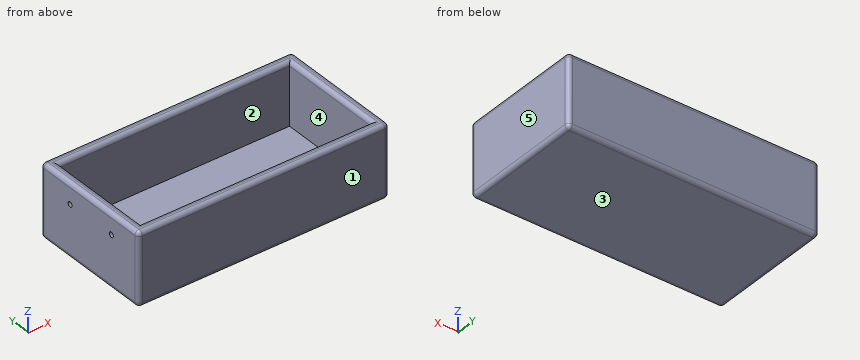
from build123d import *

# Parameters (mm, degrees)
F0_W     = 121.37
F0_H     = 60.8
F0_W_2   = 111.37
F0_H_2   = 50.8
F1_DEPTH = 5
F2_DEPTH = 35
F3_R     = 1.25
F4_DEPTH = 75
F5_R     = 2


with BuildPart() as f1:
    # F0 (on Top) → F1 (new body)
    with BuildSketch(Plane.XY):
        with Locations((-0.463949, -2.512982)):
            Rectangle(F0_W, F0_H)
        with Locations((-0.463949, -2.512982)):
            Rectangle(F0_W_2, F0_H_2, mode=Mode.SUBTRACT)
        with Locations((-0.463949, -2.512982)):
            Rectangle(F0_W_2, F0_H_2)
    extrude(amount=F1_DEPTH)

    # F0 (on Top) → F2 (join)
    with BuildSketch(Plane.XY):
        with Locations((-0.463949, -2.512982)):
            Rectangle(F0_W, F0_H)
        with Locations((-0.463949, -2.512982)):
            Rectangle(F0_W_2, F0_H_2, mode=Mode.SUBTRACT)
    extrude(amount=F2_DEPTH)

    # F3 (on Right) → F4 (cut)
    with BuildSketch(Plane.YZ):
        with Locations((-16.162982, 25.25)):
            Circle(F3_R)
        with Locations((9.637018, 25.25)):
            Circle(F3_R)
    extrude(amount=-F4_DEPTH, mode=Mode.SUBTRACT)

    # F5
    f5_edges = [f1.edges().sort_by_distance(p)[0] for p in [
        (-61.148949, -32.912982, 17.5),
        (-0.463949, -32.912982, 35),
        (60.221051, -32.912982, 17.5),
        (-0.463949, -32.912982, 0),
        (60.221051, 27.887018, 17.5),
        (-0.463949, 27.887018, 35),
        (-61.148949, 27.887018, 17.5),
        (-0.463949, 27.887018, 0),
        (60.221051, -2.512982, 35),
        (60.221051, -2.512982, 0),
        (55.221051, -2.512982, 35),
        (-0.463949, 22.887018, 35),
        (-56.148949, -2.512982, 35),
        (-0.463949, -27.912982, 35),
        (-61.148949, -2.512982, 35),
        (-61.148949, -2.512982, 0),
    ]]
    fillet(f5_edges, radius=F5_R)


solid = f1.part
The listing builds one solid part. Answer for the finished solid, in the listing's coordinates (mm). Face numbers are marked on the shaded views. A direction names the side the tool comes from. Give positions to 0.01 mm unless a question says otherwise; leave off trailing zeros. Write each loop counter-clockwise with the first axis right and the second up, starting at its lowest first coordinate (ties: lowest second). Pieces come first, ordered by that corner, then holes.
1) Given P1, Ø6, axis at x = 39.5, y = -0.5, coming from the -Z side; P2, Ø2, axis at x = -44.5, y = 0, coming from the +Z side, each flat-ended and moving along its own axis, determine where each tip first touches the part or whether it passes through.
2) Section A-A (z = 25.25) is taken. Write down the section's boundary in (x, y), and give its area (3 significant figures).
3) Find the intervals of material crossed by L1, parallel to Y at x = -58, z = 25; L2, parallel to Y at x = 12, z = 20.5; L3, parallel to X at y = -20, z = 21, in increasing order.
4) Section C-C (x = -46) is taken. Write down the section's boundary in (y, z).
5) A tool of negligible diameter and unlimited length cuts with its end or side. For the marked faces 1 and 2, from which of +Z, -Z, +X, -X, +Y, -Y can it reach the whole face along a straight path? Write none if from no direction.
6) Section B-B (y = -3.5) is taken. Write down the section's boundary in (x, z).
7) For a pull along X with two mould halves and no side action, classify the marked faces 3, 4 and 5 as pulls with the +X half, pulls with the -X half, needs draft (parallel to the pull), parting line crosses it, or undercut.
Response:
1. P1: stops at z = 0
1. P2: stops at z = 5
2. outline: (-61.15, -30.91) arc R2 ccw to (-59.15, -32.91) - (58.22, -32.91) arc R2 ccw to (60.22, -30.91) - (60.22, 25.89) arc R2 ccw to (58.22, 27.89) - (-59.15, 27.89) arc R2 ccw to (-61.15, 25.89) - (-61.15, 10.89) - (-56.15, 10.89) - (-56.15, 22.89) - (55.22, 22.89) - (55.22, -27.91) - (-56.15, -27.91) - (-56.15, -17.41) - (-61.15, -17.41) - close; (-61.15, -14.91) - (-56.15, -14.91) - (-56.15, 8.39) - (-61.15, 8.39) - close
2. area: 1,690 mm2
3. L1: y = -32.91 to -17.39, -14.94 to 8.41, 10.86 to 27.89
3. L2: y = -32.91 to -27.91, 22.89 to 27.89
3. L3: x = -61.15 to -56.15, 55.22 to 60.22
4. outline: (-32.91, 2) arc R2 ccw to (-30.91, 0) - (25.89, 0) arc R2 ccw to (27.89, 2) - (27.89, 33) arc R2 ccw to (25.89, 35) - (24.89, 35) arc R2 ccw to (22.89, 33) - (22.89, 5) - (-27.91, 5) - (-27.91, 33) arc R2 ccw to (-29.91, 35) - (-30.91, 35) arc R2 ccw to (-32.91, 33) - close
5. face 1: +Z, -Z, +X, -X, -Y
5. face 2: +Z
6. outline: (-61.15, 2) arc R2 ccw to (-59.15, 0) - (58.22, 0) arc R2 ccw to (60.22, 2) - (60.22, 33) arc R2 ccw to (58.22, 35) - (57.22, 35) arc R2 ccw to (55.22, 33) - (55.22, 5) - (-56.15, 5) - (-56.15, 33) arc R2 ccw to (-58.15, 35) - (-59.15, 35) arc R2 ccw to (-61.15, 33) - close
7. face 3: needs draft
7. face 4: undercut
7. face 5: pulls with the +X half
